```python
from build123d import *

# Parameters (mm, degrees)
F0_R     = 100
F1_DEPTH = 27
F2_R     = 15
F4_R     = 5
F5_DEPTH = 30


# Not quite as in the source:
# - a fillet or chamfer that OpenCascade refuses, or shapes differently, is made with other operations: its cross-section is extruded or revolved along the edge and cut away or added


with BuildPart() as f1:
    # F0 (on Front) → F1 (new body)
    with BuildSketch(Plane.XZ):
        Circle(F0_R)
    extrude(amount=F1_DEPTH)

    # F2
    f2_edges = [f1.edges().sort_by_distance(p)[0] for p in [
        (-100, -27, 0),
    ]]
    fillet(f2_edges, radius=F2_R)

    # F3: fillet of radius 15 on 1 edges, made by hand

    # F3_s1 → F3_t2 (revolve, cut)
    with BuildSketch(Plane.XY):
        with BuildLine():
            ThreePointArc((100, -12), (94.7898945238, -3.3810499614), (85.3030615433, 0))
            Line((85.3030615433, 0), (100, 0))
            Line((100, 0), (100, -12))
        make_face()
    revolve(axis=Axis((0, 0, 0), (0, -1, 0)), mode=Mode.SUBTRACT)

    # F4 (on face) → F5 (cut)
    with BuildSketch(Plane.XZ.offset(27)):
        Circle(F4_R)
    extrude(amount=-F5_DEPTH, mode=Mode.SUBTRACT)


solid = f1.part
```
Model file for the job. Use its own axes, mm. Round coordinates to 2 decimals unless told otherwise and drop trailing zeros. Write each loop counter-clockwise with the first axis right and the second up, starting at its lowest first coordinate (ties: lowest second). Pieces come first, ordered by that corner, then holes. Notation, with made-up numbers: M -36.75,25.5 L 10.25,25.5 A9 ccw 10.25,37.5 Z; hole C 40,12 d10. An arc over 180 degrees is marked long. Put each result on its own line as item: value.
Item 1: Cut at C-C (y = -17.25). List the corners of the cut face in (x, z), and give its area (3 significant figures).
Responses:
outline: C 0,0 d198.1; hole C 0,0 d10
area: 30,700 mm²
Item 2: Cut at A-A (z = 0). List the corners of the cut face in (x, y), and give its area (3 significant figures).
Responses:
outline: M -100,-12 A15 ccw -85,-27 L -5,-27 L -5,0 L -85.3,0 A15 ccw Z; M 5,-27 L 85,-27 A15 ccw 100,-12 A15 ccw 85.3,0 L 5,0 Z
area: 4,940 mm²
Item 3: Flat gauge pins, fed straight in: P1, Ø8, axis at x = 52.5, y = -18.5, coming from the -Z side; P2, Ø8, axis at x = -66, y = -11, coming from the +Z side; P3, Ø2, axis at x = -24, y = -14, coming from the -Z side. Where does each tip first touch, or does it go through?
Responses:
P1: z = -86.36
P2: z = 78.36
P3: z = -97.21
Item 4: Probe L1, parallel to Z at x = 0, y = -19.75; L2, parallel to Z at x = 0, y = -7.75; L3, parallel to Z at x = -44, y = -21. List the from-to ranges inside material, lowest first. Write a range as from..to.
Responses:
L1: -97.84..-5, 5..97.84
L2: -98.43..-5, 5..98.43
L3: -86.45..86.45
Item 5: Cut at B-B (x = 0). List the corners of the cut face in (y, z), and give its area (3 significant figures).
Responses:
outline: M -27,-85 A15 ccw -12,-100 A15 ccw 0,-85.3 L 0,-5 L -27,-5 Z; M -27,5 L 0,5 L 0,85.3 A15 ccw -12,100 A15 ccw -27,85 Z
area: 4,940 mm²
Item 6: Mould opens along X. For faces 1 (the cylindrical face through (-1.08, -13.69, -4.88)), 2 (the flat face through (-1, 0, -18)) say: +X half, -X half, draft (parallel to the pull), parting line (faces both ways), or undercut.
Responses:
face 1: undercut
face 2: draft
